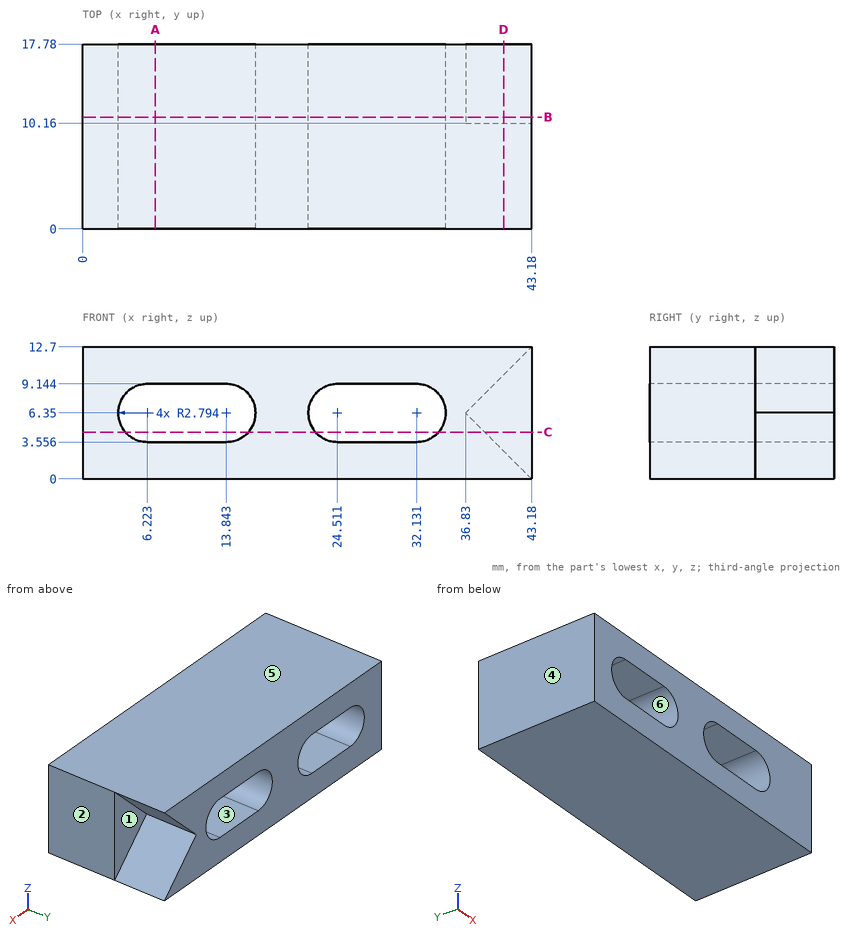
Here's the drawing with two shaded views (mm, measured from the low corner). I have some questions. A direction names the side the tool comes from. Give positions to 0.01 mm unless a question says otherwise; leave off trailing zeros. Order: outer loops, then holes, each group sorted by start corner. A loop starts at its lowest first (then second) coordinate and runs counter-clockwise, first axis right, second up.
Q1. We'd pull the mould along Z, two halves only. Please class the marked faces 4, 5 and 6: +Z half, -Z half, draft (parallel to the pull), parting line (faces both ways), or undercut.
Q2. Suppose I cut it at B-B, the plane y = 10.75. Write out the boundary of the cut face in (x, z).
Q3. For the marked faces 1, 2 and 3, which set-ups out of +Z, -Z, +X, -X, +Y, -Y let a thin tool reach every point of the face, with its end or its side?
Q4. Suppose I cut it at D-D, the plane x = 40.5. Write out the boundary of the cut face in (y, z), and give its area (3 significant figures).
Q5. Suppose I cut it at C-C, the plane z = 4.5. Write out the boundary of the cut face in (x, y).
Q6. Suppose I cut it at A-A, the plane x = 7. Write out the boundary of the cut face in (y, z).
Q7. If I drill on line 1 along X through (y, z) = (14.25, 6.75); line 2 along X through (y, z) = (11, 5); line 3 along Z through (x, y) = (8, 11.75), over which ranges is the centre line in solid material (lowest first)?
Q8. I'm going to push a flat-ended pin straight in: P1, Ø1.5, axis at y = 13, z = 9, coming from the +X side. Where does the tip first touch, or does it pass through?
Solution:
1. face 4: draft
1. face 5: +Z half
1. face 6: undercut
2. outline: (0, 0) - (43.18, 0) - (36.83, 6.35) - (43.18, 12.7) - (0, 12.7) - close; hole (6.22, 3.56) - (13.84, 3.56) arc R2.79 ccw to (13.84, 9.14) - (6.22, 9.14) arc R2.79 ccw to start; hole (24.51, 3.56) - (32.13, 3.56) arc R2.79 ccw to (32.13, 9.14) - (24.51, 9.14) arc R2.79 ccw to start
3. face 1: +X, +Y
3. face 2: +Z, -Z, +X, +Y, -Y
3. face 3: +Y, -Y
4. outline: (0, 0) - (17.78, 0) - (17.78, 2.68) - (10.16, 2.68) - (10.16, 10.02) - (17.78, 10.02) - (17.78, 12.7) - (0, 12.7) - close
4. area: 170 mm2
5. outline: (0, 0) - (4.13, 0) - (4.13, 17.78) - (0, 17.78) - close; (15.94, 0) - (22.42, 0) - (22.42, 17.78) - (15.94, 17.78) - close; (34.22, 0) - (43.18, 0) - (43.18, 10.16) - (38.68, 10.16) - (38.68, 17.78) - (34.22, 17.78) - close
6. outline: (0, 0) - (17.78, 0) - (17.78, 3.56) - (0, 3.56) - close; (0, 9.14) - (17.78, 9.14) - (17.78, 12.7) - (0, 12.7) - close
7. line 1: x = 0 to 3.46, 16.61 to 21.75, 34.9 to 37.23
7. line 2: x = 0 to 3.78, 16.29 to 22.06, 34.58 to 38.18
7. line 3: z = 0 to 3.56, 9.14 to 12.7
8. P1: stops at x = 40.23
